Autodesk Inventor part; units mm, degrees
ref_plane "YZ Plane" through (0, 0, 0) normal (1, 0, 0) x (0, 1, 0)
ref_plane "XZ Plane" through (0, 0, 0) normal (0, 1, 0) x (-1, 0, 0)
ref_plane "XY Plane" through (0, 0, 0) normal (0, 0, 1) x (1, 0, 0)
sketch "Skizze1" plane through (0, 0, 0) normal (0, 0, 1) x (1, 0, 0)
  line L0 (-6, 0) -> (1, 0)
  line L1 (0, -1) -> (0, 6)
  line L2 (0, 0) -> (0, 5)
  line L3 (0, 5) -> (-1.5, 5)
  line L4 (-1.5, 5) -> (-1.5, 3.5)
  line L5 (-1.5, 3.5) -> (-2.5, 3.5)
  line L6 (-2.5, 3.5) -> (-3, 4)
  line L7 (-3, 4) -> (-5, 4)
  line L8 (-5, 4) -> (-5, 0)
  line L9 (-5, 0) -> (0, 0)
  dimension "d0" = 8
  dimension "d1" = 10
  dimension "d2" = 1.5
  dimension "d3" = 1
  dimension "d4" = 7
  dimension "d5" = 45
  dimension "d6" = 5
revolve "Umdrehung1" add sketch "Skizze1" angle 360 about axis through (-10, 0, 0) along (1, 0, 0)
sketch "Skizze2" plane through (0, 0, 0) normal (1, 0, 0) x (0, 0, -1)
  line L0 (-7.1847, 0.5) -> (7.4374, 0.5)
  line L1 (7.4374, 0.5) -> (7.4374, -0.5)
  line L2 (7.4374, -0.5) -> (-7.1847, -0.5)
  line L3 (-7.1847, -0.5) -> (-7.1847, 0.5)
  line L4 (0, -7) -> (0, 7)
  line L5 (10.3619, 0) -> (-10.1091, 0)
  dimension "d8" = 1
extrude "Extrusion1" cut sketch "Skizze2" against normal blind 1
thread "Gewinde1"
chamfer "Fase1" distance 0.5 angle 45 3 edges at (0, -5, 0) (0, 3.7081, -3.3541) (0, 3.7081, 3.3541)
properties part number "13_1087_042"
The listing builds one solid part. Answer for the finished solid, in the listing's coordinates (mm). A direction names the side the tool comes from. Coordinates: 2 decimals unless noted, no trailing zeros. Write each loop counter-clockwise with the first axis right and the second up, starting at its lowest first coordinate (ties: lowest second). Pieces come first, ordered by that corner, then holes. Notation, with made-up numbers: (27.5, -0.5) - (32.5, -0.5) arc R5 cw to (32.5, 6.5) - close; hole circle Ø11 at (79, -27.75). An arc over 180 degrees is marked (long way). Return JSON: item names as keys, results as strings. Group by question number.
Q1. The part is cut by section B-B on y = 0. Write down the section's boundary in (x, z).
Q2. Find the intervals of material crossed by line 1 along Y through (x, z) = (-0.3, 3); line 2 along Y through (x, z) = (-0.3, -1.75); line 3 along X through (y, z) = (0.75, -3.75), in increasing order. Write a range as [from, to].
Q3. For a pull along X with two mould halves and no side action, classify faces 5 (the conical face through (-0.14, -4.64, -0.1)), 6 (the flat face through (-1.5, 2.2, -3.3)), 7 (the flat face through (-5, 0, 0)) as +X half, -X half, draft (parallel to the pull), parting line (faces both ways), or undercut.
Q4. The part is cut by section A-A on z = 0. Write down the section's boundary in (x, y), and give its area (3 significant figures).
Q5. The part is cut by section D-D on x = -4.4. Write down the section's boundary in (y, z).
Q6. Which of the six approach directions +Z, -Z, +X, -X, +Y, -Y give full straight-line access (tool end or side, diameter ignored) to faces 1 (the cylindrical face through (-2.007, 3.233, 1.341)), 2 (the conical face through (-0.14, 4.64, 0.1)), 3 (the flat face through (-0.5, 0.5, 0.1)), 4 (the cylindrical face through (-4.014, -0.867, 3.905))?
Q7. The part is cut by section C-C on x = -2.85. Write down the section's boundary in (y, z).
Q8. Flat-ended cylindrical pins translate along their axes: pin 1 Ø1 at (x, z) = (-2.5, -1) entering from +Y; pin 2 Ø2 at (x, y) = (-2, -3.5) entering from -Z; pin 3 Ø0.5 at (x, z) = (-0.5, 1) entering from -Y. Find the tip coordinate at first contact, or state that the pin passes through.
Evaluation:
{
 "1": {"outline": "(-5, -4) - (-3, -4) - (-2.5, -3.5) - (-1.5, -3.5) - (-1.5, -5) - (-1, -5) - (-1, 5) - (-1.5, 5) - (-1.5, 3.5) - (-2.5, 3.5) - (-3, 4) - (-5, 4) - close"},
 "2": {"line 1": "y = [-3.75, -0.5], [0.5, 3.75]", "line 2": "y = [-4.47, -0.5], [0.5, 4.47]", "line 3": "x = [-5, -2.82], [-1.5, 0]"},
 "3": {"face 5": "+X half", "face 6": "undercut", "face 7": "-X half"},
 "4": {"outline": "(-5, -4) - (-3, -4) - (-2.5, -3.5) - (-1.5, -3.5) - (-1.5, -5) - (-0.5, -5) - (0, -4.5) - (0, -0.5) - (-1, -0.5) - (-1, 0.5) - (0, 0.5) - (0, 4.5) - (-0.5, 5) - (-1.5, 5) - (-1.5, 3.5) - (-2.5, 3.5) - (-3, 4) - (-5, 4) - close", "area": "40.5 mm2"},
 "5": {"outline": "circle Ø8 at (0, 0)"},
 "6": {"face 1": "none", "face 2": "+X, +Y", "face 3": "+Z, -Z, +X", "face 4": "-X"},
 "7": {"outline": "circle Ø7.7 at (0, 0)"},
 "8": {"pin 1": "stops at y = 3.89", "pin 2": "stops at z = -4.25", "pin 3": "stops at y = -4.94"}
}
